Could you check a few things on this model? Use its own coordinates, in mm. Face numbers are marked on the shaded views. Give positions to 0.01 mm unless a question says otherwise; leave off trailing zeros. Loops run counter-clockwise (first coordinate to the right, second up) from the corner with the lowest first, then second, coordinate; pieces in that order, holes last. Notation, with made-up numbers: (49.25, 24.5) - (81.25, 24.5) arc R34 ccw to (81.25, 55.5) - close; hole circle Ø7 at (10, -32.75). An arc over 180 degrees is marked (long way). Write each question's results on one line, items separated by ' | '. Start each with the question number.
```python
from build123d import *

# Parameters (mm, degrees)
BOSS_EXTRUDE1_DEPTH     = 1321.809345804
BOSS_EXTRUDE2_DEPTH     = 110
BOSS_EXTRUDE4_DEPTH     = 80
CUT_EXTRUDE1_DEPTH      = 390
CUT_EXTRUDE1_DEPTH_BACK = 1710
SKETCH4_R               = 10.935754795
SKETCH4_R_2             = 10.805085865
CUT_EXTRUDE2_DEPTH      = 10
CUT_EXTRUDE2_DEPTH_BACK = 1600
CUT_EXTRUDE3_DEPTH      = 1600
CUT_EXTRUDE3_DEPTH_BACK = 1800
SKETCH7_W               = 1261.809345804
SKETCH7_H               = 148.826585301


with BuildPart() as part:
    # Sketch1 → Boss-Extrude1 (new body)
    with BuildSketch(Plane(origin=(0, 0, 0), x_dir=(0, 0, -1), z_dir=(1, 0, 0))):
        Polygon((0, 0), (1214.174590511, 618.652853995), (1188.297132026, 669.440225874), (-25.877458485, 50.787371879), (-460.955944246, -170.896189144), (-435.078485761, -221.683561023), align=None)
    extrude(amount=-BOSS_EXTRUDE1_DEPTH)

    # Sketch2 → Boss-Extrude2 (add)
    with BuildSketch(Plane(origin=(0, 50.787371879, 25.877458485), x_dir=(1, 0, 0), z_dir=(0, 0.8910065241883673, 0.453990499739548))):
        Polygon((0, 0), (0, -488.3), (-67.842597561, -488.3), (-67.842597561, 0), (-67.842597561, 1244.513029496), (0, 1244.513029496), align=None)
        Polygon((-1321.809345804, 0), (-1321.809345804, 1244.513029496), (-1253.966748243, 1244.513029496), (-1253.966748243, 0), (-1253.966748243, -488.3), (-1321.809345804, -488.3), align=None)
    extrude(amount=BOSS_EXTRUDE2_DEPTH)

    # Sketch3 → Boss-Extrude4 (add)
    with BuildSketch(Plane.ZY.offset(1321.809345804)):
        Polygon((-882.563635412, 626.858827585), (-795.042959323, 580.236826077), (-834.961493519, 505.300165527), (-922.482169607, 551.922167035), align=None)
        Polygon((-41.133790816, 178.631674443), (41.227375134, 134.758128502), (9.982813434, 76.104594213), (-72.378352516, 119.978140155), align=None)
    extrude(amount=BOSS_EXTRUDE4_DEPTH)

    # Sketch4 → Cut-Extrude1 (cut, two sides: drawn at the far end of the back side and taken through both)
    with BuildSketch(Plane(origin=(0, 0, 0), x_dir=(0, 0, -1), z_dir=(1, 0, 0)).offset(-CUT_EXTRUDE1_DEPTH_BACK)):
        with Locations(Location((19.453016292, 135.017213441, 0), (0, 0, 180))):
            Circle(SKETCH4_R)
        with Locations(Location((863.462816879, 576.936245259, 0), (0, 0, 180))):
            Circle(SKETCH4_R_2)
    extrude(amount=CUT_EXTRUDE1_DEPTH + CUT_EXTRUDE1_DEPTH_BACK, mode=Mode.SUBTRACT)

    # Sketch5 → Cut-Extrude2 (cut, two sides: drawn at the far end of the back side and taken through both)
    with BuildSketch(Plane(origin=(0, 0, 0), x_dir=(0, 0, -1), z_dir=(1, 0, 0)).offset(-CUT_EXTRUDE2_DEPTH_BACK)):
        Polygon((1033.052815262, 713.795181733), (1054.736624804, 671.238309325), (949.530250393, 671.238309325), align=None)
    extrude(amount=CUT_EXTRUDE2_DEPTH + CUT_EXTRUDE2_DEPTH_BACK, mode=Mode.SUBTRACT)

    # Sketch7 → Cut-Extrude3 (cut, two sides: drawn at the far end of the back side and taken through both)
    with BuildSketch(Plane(origin=(0, -221.683561023, 435.078485761), x_dir=(1, 0, 0), z_dir=(0, -0.453990499739547, 0.8910065241883678)).offset(-CUT_EXTRUDE3_DEPTH_BACK)):
        with Locations((-660.904672902, 131.413292651)):
            Rectangle(SKETCH7_W, SKETCH7_H)
    extrude(amount=CUT_EXTRUDE3_DEPTH + CUT_EXTRUDE3_DEPTH_BACK, mode=Mode.SUBTRACT)


solid = part.part
```
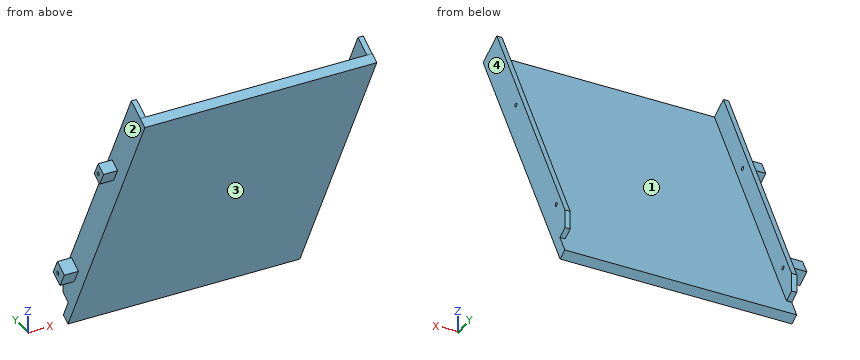
Q1. I'm going to push flat-ended pins straight in: pin 1 Ø4 at (x, y) = (-667, 146) entering from +Z; pin 2 Ø4 at (x, z) = (-957.5, -538.5) entering from +Y; pin 3 Ø5 at (y, z) = (239, -111) entering from -X. Where does each tip first touch, or does it pass through?
Q2. I need wall thicknesses on L1, parallel to X at y = -76.5, z = 329.5; L2, parallel to Y at x = -832.5, z = -0.5; L3, parallel to Z at x = -843, y = 457.5. Which ranges of each line are inside material? Lowest first, please. Write a range as from..to.
Q3. I want a section at C-C, the plane x = -196. List the corners of the cut face in (y, z) for me.
Q4. I want a section at B-B, the plane y = 408. List the corners of the cut face in (x, z) for me.
Q5. I want a section at A-A, the plane z = -1029.5. List the corners of the cut face in (x, y) for me.
Q6. If we mould it in two halves opening along X, with no side actions, what happens to the marked faces 1, 2, 3 and 4? For each: +X half, -X half, draft (parallel to the pull), parting line (faces both ways), or undercut.
Conclusion:
1) pin 1: z = -157.06 | pin 2: y = 339.37 | pin 3: x = -1321.81
2) L1: -1321.81..-1291.81, -30..0 | L2: 0.25..64.23 | L3: -897.89..-772.34
3) outline: (-221.68, 435.08) - (618.65, -1214.17) - (669.44, -1188.3) - (-170.9, 460.96) - close
4) outline: (-1321.81, -800.75) - (0, -800.75) - (0, -432.9) - (-30, -432.9) - (-30, -675.19) - (-1291.81, -675.19) - (-1291.81, -432.9) - (-1321.81, -432.9) - close
5) outline: (-1321.81, 524.56) - (0, 524.56) - (0, 671.24) - (-30, 671.24) - (-30, 588.53) - (-1291.81, 588.53) - (-1291.81, 671.24) - (-1321.81, 671.24) - close
6) face 1: undercut | face 2: -X half | face 3: draft | face 4: +X half
